from build123d import *

# Parameters (mm, degrees)
F0_R     = 6.35
F1_DEPTH = 3.175


with BuildPart() as f1:
    # F0 (on Front) → F1 (new body)
    with BuildSketch(Plane.XZ):
        with BuildLine():
            ThreePointArc((0, 25.4), (-25.287129, -2.391879), (4.7625, -24.949521))
            ThreePointArc((4.7625, -24.949521), (19.572014, -16.189387), (25.4, 0))
            ThreePointArc((25.4, 0), (17.960512, 17.960512), (0, 25.4))
        make_face()
        Circle(F0_R, mode=Mode.SUBTRACT)
        with BuildLine():
            Line((-95.035584, -43.999521), (4.7625, -24.949521))
            ThreePointArc((4.7625, -24.949521), (-25.287129, -2.391879), (0, 25.4))
            ThreePointArc((0, 25.4), (-24.225165, 43.164465), (-14.564732, 71.609339))
            Line((-14.564732, 71.609339), (-114.362815, 1.759339))
            ThreePointArc((-114.362815, 1.759339), (-88.067444, 3.478917), (-74.398084, -19.05))
            ThreePointArc((-74.398084, -19.05), (-80.226069, -35.239387), (-95.035584, -43.999521))
        make_face()
        with BuildLine():
            ThreePointArc((0, 25.4), (17.960512, 17.960512), (25.4, 0))
            Line((25.4, 0), (25.4, 50.8))
            ThreePointArc((25.4, 50.8), (17.960512, 32.839488), (0, 25.4))
        make_face()
        with BuildLine():
            ThreePointArc((-14.564732, 71.609339), (-24.225165, 43.164465), (0, 25.4))
            ThreePointArc((0, 25.4), (17.960512, 32.839488), (25.4, 50.8))
            ThreePointArc((25.4, 50.8), (11.73064, 73.328917), (-14.564732, 71.609339))
        make_face()
        with BuildLine():
            ThreePointArc((-10.991184, 43.071134), (-18.815754, 47.478073), (-14.408816, 55.302643))
            ThreePointArc((-14.408816, 55.302643), (0, 57.277815), (14.408816, 55.302643))
            ThreePointArc((14.408816, 55.302643), (17.758334, 53.025607), (19.05, 49.186888))
            ThreePointArc((19.05, 49.186888), (16.538719, 44.128555), (10.991184, 43.071134))
            ThreePointArc((10.991184, 43.071134), (0, 44.577815), (-10.991184, 43.071134))
        make_face(mode=Mode.SUBTRACT)
        with BuildLine():
            ThreePointArc((-114.362815, 1.759339), (-123.196572, -28.932851), (-95.035584, -43.999521))
            ThreePointArc((-95.035584, -43.999521), (-80.226069, -35.239387), (-74.398084, -19.05))
            ThreePointArc((-74.398084, -19.05), (-88.067444, 3.478917), (-114.362815, 1.759339))
        make_face()
        with Locations((-99.798084, -19.05)):
            Circle(F0_R, mode=Mode.SUBTRACT)
    extrude(amount=F1_DEPTH)


solid = f1.part
For this review, take the finished solid that the model builds, in its own axes (mm). A direction names the side the tool comes from. Round coordinates to 2 decimals unless told otherwise and drop trailing zeros. Loops run counter-clockwise (first coordinate to the right, second up) from the corner with the lowest first, then second, coordinate; pieces in that order, holes last. Notation, with made-up numbers: (-10, 55.25) - (1, 55.25) arc R31 ccw to (1, 79.25) - close; hole circle Ø2 at (-21, -20.5). An arc over 180 degrees is marked (long way). Put each result on its own line as item: value. Start each with the question number.
1. For faces 4 (the flat face through (-45.8, -1.6, -34.6)), 5 (the cylindrical face through (-0.204, -1.565, 57.277)), list the 3-axis set-ups (+Z, -Z, +X, -X, +Y, -Y) from which the entire face can be reached by the end or side of a thin tool; tool diameter is ignored.
2. Consider section A-A on y = -2.3. State the section outline as (x, z) points.
3. For probe 1 along Z at (x, y) = (0, -1.7); probe 2 along X at (y, z) = (-2.65, 2); probe 3 along Z at (x, y) = (-13.5, -0.65), list the stretches that pass through material, from the lowest coordinate up. Write a range as [from, to].
4. Consider section B-B on x = 0. State the section outline as (y, z) points (3 decimals), plus the area to 3 significant figures.
5. Mouldability with a two-part tool opening along Z and no side actions: class faces 1 (the cylindrical face through (-93.93, -1.57, -21.48)), 2 (the cylindrical face through (-123.38, -1.57, -28.49)), 3 (the flat face through (-34, -3.175, 3)) as +Z half, -Z half, draft (parallel to the pull), parting line (faces both ways), or undercut.
6. Consider section D-D on z = 35.5. State the section outline as (x, y) points (3 decimals), plus the area to 3 significant figures.
7. Consider section C-C on z = -15. State the section outline as (x, y) points (3 decimals).
Result sheet:
1. face 4: -Z, +X, +Y, -Y
1. face 5: +Y, -Y
2. outline: (-114.36, 1.76) arc R25.4 ccw to (-95.04, -44) - (4.76, -24.95) arc R25.4 ccw to (25.4, 0) - (25.4, 50.8) arc R25.4 ccw to (-14.56, 71.61) - close; hole circle Ø12.7 at (-99.8, -19.05); hole (-14.41, 55.3) arc R6.35 ccw to (-10.99, 43.07) arc R40.84 cw to (10.99, 43.07) arc R6.35 ccw to (14.41, 55.3) arc R53.54 ccw to start; hole circle Ø12.7 at (0, 0)
3. probe 1: [-25.86, -6.35], [6.35, 44.58], [57.28, 76.2]
3. probe 2: [-114.02, -6.03], [6.03, 25.4]
3. probe 3: [-28.44, 42.89], [55.55, 72.32]
4. outline: (-3.175, -25.859) - (0, -25.859) - (0, -6.35) - (-3.175, -6.35) - close; (-3.175, 6.35) - (0, 6.35) - (0, 44.578) - (-3.175, 44.578) - close; (-3.175, 57.278) - (0, 57.278) - (0, 76.2) - (-3.175, 76.2) - close
4. area: 243 mm^2
5. face 1: undercut
5. face 2: parting line
5. face 3: draft
6. outline: (-66.156, -3.175) - (25.4, -3.175) - (25.4, 0) - (-66.156, 0) - close
6. area: 291 mm^2
7. outline: (-124.873, -3.175) - (-104.689, -3.175) - (-104.689, 0) - (-124.873, 0) - close; (-94.907, -3.175) - (20.498, -3.175) - (20.498, 0) - (-94.907, 0) - close
